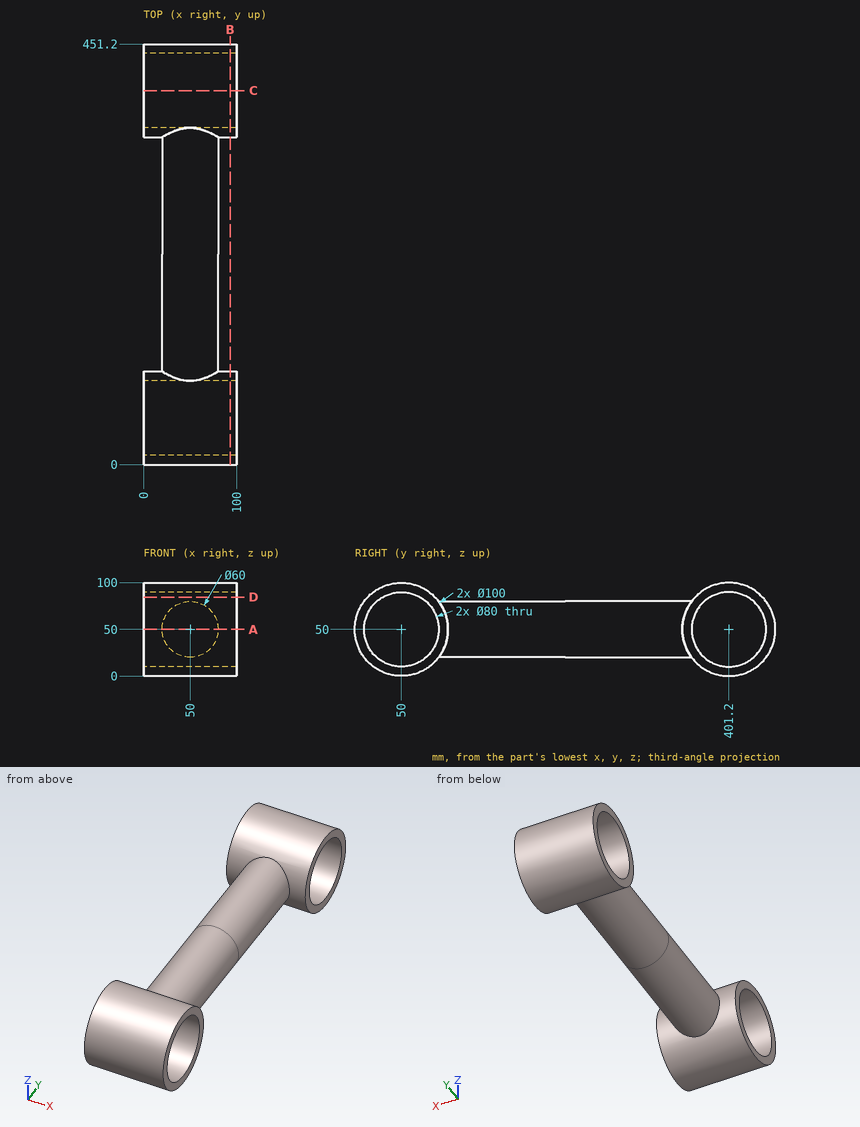
Source: three-view drawing plus pictorial views. Frame: mm from the lowest corner of the part. Round coordinates to 2 decimals unless told otherwise and drop trailing zeros. Loops run counter-clockwise (first coordinate to the right, second up) from the corner with the lowest first, then second, coordinate; pieces in that order, holes last. Notation, with made-up numbers: (-24, 33) - (18, 33) arc R16 cw to (18, 45) - close; hole circle Ø1 at (68, 0). An arc over 180 degrees is marked (long way). Write each question's results on one line, items separated by ' | '. Start each with the question number.
1) Cut plane D-D on z = 84.5. Return loops of the section in (x, y).
2) Cut plane B-B on x = 93. Return loops of the section in (y, z), then the cut area to 3 significant figures.
3) Line query: probe 1 along Y at (x, z) = (62, 50); probe 2 along Y at (x, z) = (70.5, 19); probe 3 along Y at (x, z) = (22.5, 32). Output: solid intervals per line, ascending. Write a range as [from, to].
4) Cut plane A-A on z = 50. Return loops of the section in (x, y), then the cut area to 3 significant figures.
5) First-contact query: P1, Ø3, axis at x = 47.5, y = 240, coming from the -Z side; P2, Ø1.5, axis at y = 107, z = 41.5, coming from the +X side; P3, Ø6, axis at x = 72, z = 55, coming from the +Y side. Flat tips, straight axial feed; report the tip coordinate or a pass-through.
6) Cut plane C-C on y = 401.2. Return loops of the section in (x, z).
Verdict:
1) outline: (0, 13.81) - (100, 13.81) - (100, 29.76) - (0, 29.76) - close; (0, 70.24) - (100, 70.24) - (100, 86.19) - (0, 86.19) - close; (0, 365.01) - (100, 365.01) - (100, 380.96) - (0, 380.96) - close; (0, 421.44) - (100, 421.44) - (100, 437.39) - (0, 437.39) - close
2) outline: circle Ø100 at (50, 50); circle Ø100 at (401.2, 50); hole circle Ø80 at (50, 50); hole circle Ø80 at (401.2, 50) | area: 5,650 mm2
3) probe 1: y = [0, 10], [90, 361.2], [441.2, 451.2] | probe 2: y = [10.77, 24.72], [75.28, 89.23], [361.97, 375.92], [426.48, 440.43] | probe 3: y = [3.35, 14.28], [85.72, 96.65], [354.55, 365.48], [436.92, 447.85]
4) outline: (0, 0) - (100, 0) - (100, 10) - (0, 10) - close; (0, 90) - (100, 90) - (100, 100) - (80, 100) - (80, 351.2) - (100, 351.2) - (100, 361.2) - (0, 361.2) - (0, 351.2) - (20, 351.2) - (20, 100) - (0, 100) - close; (0, 441.2) - (100, 441.2) - (100, 451.2) - (0, 451.2) - close | area: 19,100 mm2
5) P1: stops at z = 20.02 | P2: stops at x = 78.98 | P3: stops at y = 451.16
6) outline: (0, 0) - (100, 0) - (100, 10) - (0, 10) - close; (0, 90) - (100, 90) - (100, 100) - (0, 100) - close
